Here's how the part is built. I have some questions about the finished solid (model axes, mm). A direction names the side the tool comes from. Coordinates: 2 decimals unless noted, no trailing zeros. Write each loop counter-clockwise with the first axis right and the second up, starting at its lowest first coordinate (ties: lowest second). Pieces come first, ordered by that corner, then holes.
```python
from build123d import *

# Parameters (mm, degrees)
SKETCH_1_R                  = 100
SKETCH_1_W                  = 200
SKETCH_1_H                  = 40
EXTRUDE_524_DEPTH           = 3
SKETCH_3_W                  = 30
SKETCH_3_H                  = 40
SKETCH_3_W_2                = 20
SKETCH_3_H_2                = 30
SKETCH_3_H_3                = 10
CUT_EXTRUDE_1393_DEPTH      = 3
SKETCH_2_R                  = 2
SKETCH_2_R_2                = 1.5
CUT_EXTRUDE_2567_DEPTH      = 173.072659072
REVOLVE_3158_ANGLE          = 90
EXTRUDE_3359_DEPTH          = 40
SKETCH_8_W                  = 10
SKETCH_8_H                  = 8
EXTRUDE_L_DEPTH             = 100
EXTRUDE_L_32_DEPTH          = 10
SKETCH_16_W                 = 2
SKETCH_16_H                 = 84
CUT_EXTRUDE_L_DEPTH         = 5
SKETCH_23_W                 = 200
SKETCH_23_H                 = 3
EXTRUDE_5603_DEPTH          = 100
CUT_EXTRUDE_5983_DEPTH      = 100
CUT_EXTRUDE_5983_DEPTH_BACK = 100
CUT_EXTRUDE_6828_DEPTH      = 100


# Read off the part's stored shape, not the designer's step: the extrude step
with BuildPart() as part:
    # Sketch 1 → Extrude 524 (new body)
    with BuildSketch(Plane(origin=(0, 0, 0), x_dir=(1, 0, 0), z_dir=(0, 1, 0))):
        Circle(SKETCH_1_R)
        with Locations((0, 40)):
            Circle(SKETCH_1_R)
        with Locations((0, 20)):
            Rectangle(SKETCH_1_W, SKETCH_1_H)
    extrude(amount=EXTRUDE_524_DEPTH)

    # Sketch 3 → Cut-Extrude 1393 (cut)
    with BuildSketch(Plane(origin=(0, 3, 0), x_dir=(1, 0, 0), z_dir=(0, 1, 0))):
        with Locations((-79, 20)):
            Rectangle(SKETCH_3_W, SKETCH_3_H)
        with Locations((79, 20)):
            Rectangle(SKETCH_3_W, SKETCH_3_H)
        with Locations((0, -52)):
            Rectangle(SKETCH_3_W_2, SKETCH_3_H_2)
        with Locations((-45, 65)):
            Rectangle(SKETCH_3_W_2, SKETCH_3_H_3)
        with Locations((45, 65)):
            Rectangle(SKETCH_3_W_2, SKETCH_3_H_3)
    extrude(amount=-CUT_EXTRUDE_1393_DEPTH, mode=Mode.SUBTRACT)

    # Sketch 2 → Cut-Extrude 2567 (cut, through all)
    with BuildSketch(Plane(origin=(0, 3, 0), x_dir=(1, 0, 0), z_dir=(0, 1, 0))):
        with Locations(Location((-88, 66, 0), (0, 0, 270))):
            Circle(SKETCH_2_R)
        with Locations(Location((-26, 66, 0), (0, 0, 270))):
            Circle(SKETCH_2_R)
        with Locations(Location((-26, 114, 0), (0, 0, 270))):
            Circle(SKETCH_2_R)
        with Locations(Location((26, 114, 0), (0, 0, 270))):
            Circle(SKETCH_2_R)
        with Locations(Location((26, 66, 0), (0, 0, 270))):
            Circle(SKETCH_2_R)
        with Locations(Location((88, 66, 0), (0, 0, 270))):
            Circle(SKETCH_2_R)
        with Locations(Location((-45, -22, 0), (0, 0, 270))):
            Circle(SKETCH_2_R)
        with Locations(Location((45, -22, 0), (0, 0, 270))):
            Circle(SKETCH_2_R)
        with Locations(Location((-40, -82, 0), (0, 0, 270))):
            Circle(SKETCH_2_R)
        with Locations(Location((40, -82, 0), (0, 0, 270))):
            Circle(SKETCH_2_R)
        with Locations(Location((-45, 90, 0), (0, 0, 270))):
            Circle(SKETCH_2_R_2)
        with Locations(Location((45, 90, 0), (0, 0, 270))):
            Circle(SKETCH_2_R_2)
    extrude(amount=-CUT_EXTRUDE_2567_DEPTH, mode=Mode.SUBTRACT)

    # Sketch 18 → Revolve 3158 (revolve)
    with BuildSketch(Plane(origin=(0, 3, 0), x_dir=(1, 0, 0), z_dir=(0, 1, 0))):
        with BuildLine():
            Line((-97, 0), (-100, 0))
            ThreePointArc((-100, 0), (0, -100), (100, 0))
            Line((100, 0), (97, 0))
            ThreePointArc((97, 0), (0, -97), (-97, 0))
        make_face()
    revolve(axis=Axis((-100, 3, 0), (-1, 0, 0)), revolution_arc=REVOLVE_3158_ANGLE)

    # Sketch 19 → Extrude 3359 (add)
    with BuildSketch(Plane(origin=(0, 0, 0), x_dir=(-1, 0, 0), z_dir=(0, 0, -1))):
        with BuildLine():
            Line((97, 3), (100, 3))
            ThreePointArc((100, 3), (0, 103), (-100, 3))
            Line((-100, 3), (-97, 3))
            ThreePointArc((-97, 3), (0, 100), (97, 3))
        make_face()
    extrude(amount=EXTRUDE_3359_DEPTH)

    # Sketch 8 → Extrude L (add)
    with BuildSketch(Plane(origin=(0, 3, 0), x_dir=(1, 0, 0), z_dir=(0, 1, 0))):
        with Locations((-55, 0)):
            Rectangle(SKETCH_8_W, SKETCH_8_H)
    extrude_l = extrude(amount=EXTRUDE_L_DEPTH)

    # Sketch 11 → Extrude L-32 (add)
    with BuildSketch(Plane.ZY.offset(60)):
        Polygon((37, 3), (4, 60.15767665), (3.758069686, 76.576712245), (46.237604307, 3), align=None)
    extrude_l_32 = extrude(amount=-EXTRUDE_L_32_DEPTH)

    # Sketch 16 → Cut-Extrude L (cut)
    with BuildSketch(Plane(origin=(-50, 0, 0), x_dir=(0, 0, -1), z_dir=(1, 0, 0))):
        Polygon((-32.464101615, 16.856406461), (-34.196152423, 17.856406461), (15.803847577, 104.458946839), (17.535898385, 103.458946839), align=None)
        with Locations((0, 61)):
            Rectangle(SKETCH_16_W, SKETCH_16_H)
    cut_extrude_l = extrude(amount=-CUT_EXTRUDE_L_DEPTH, mode=Mode.SUBTRACT)

    # Mirror R: Extrude L, Extrude L-32, Cut-Extrude L across plane
    add(extrude_l.mirror(Plane(origin=(0, 0, 0), x_dir=(0, 0, 1), z_dir=(1, 0, 0))))
    add(extrude_l_32.mirror(Plane(origin=(0, 0, 0), x_dir=(0, 0, 1), z_dir=(1, 0, 0))))
    add(cut_extrude_l.mirror(Plane(origin=(0, 0, 0), x_dir=(0, 0, 1), z_dir=(1, 0, 0))), mode=Mode.SUBTRACT)

    # Sketch 23 → Extrude 5603 (add)
    with BuildSketch(Plane(origin=(0, 3, 0), x_dir=(1, 0, 0), z_dir=(0, 1, 0))):
        with Locations((0, 41.5)):
            Rectangle(SKETCH_23_W, SKETCH_23_H)
    extrude(amount=EXTRUDE_5603_DEPTH)

    # Sketch 24 → Cut-Extrude 5983 (cut, two sides: drawn at the far end of the back side and taken through both)
    with BuildSketch(Plane.XY.offset(-40).offset(-CUT_EXTRUDE_5983_DEPTH_BACK)):
        with BuildLine():
            ThreePointArc((0, 153), (-106.066017178, 109.066017178), (-150, 3))
            Line((-150, 3), (-100, 3))
            ThreePointArc((-100, 3), (-70.710678119, 73.710678119), (0, 103))
            Line((0, 103), (100, 103))
            Line((100, 103), (100, 3))
            Line((100, 3), (150, 3))
            ThreePointArc((150, 3), (106.066017178, 109.066017178), (0, 153))
        make_face()
        with BuildLine():
            Line((100, 3), (100, 103))
            Line((100, 103), (0, 103))
            ThreePointArc((0, 103), (70.710678119, 73.710678119), (100, 3))
        make_face()
    extrude(amount=CUT_EXTRUDE_5983_DEPTH + CUT_EXTRUDE_5983_DEPTH_BACK, mode=Mode.SUBTRACT)

    # Cut-Extrude 6828 outline → Cut-Extrude 6828 (cut)
    with BuildSketch(Plane(origin=(0, 3, 0), x_dir=(1, 0, 0), z_dir=(0, 1, 0))):
        with BuildLine():
            Line((50, 43), (-50, 43))
            Line((-50, 43), (-50, -50))
            ThreePointArc((-50, -50), (0, -70.710678119), (50, -50))
            Line((50, -50), (50, 43))
        make_face()
    extrude(amount=CUT_EXTRUDE_6828_DEPTH, mode=Mode.SUBTRACT)


solid = part.part
```
1) Imagine slicing it at B-B on z = 17. Please give me the cut outline in (x, y).
Values follow:
outline: (-98.54, 0) - (98.54, 0) - (98.54, 3) arc R98.54 ccw to (50, 87.92) - (50, 84.36) arc R95.5 cw to (95.5, 3) - (-95.5, 3) arc R95.5 cw to (-50, 84.36) - (-50, 87.92) arc R98.54 ccw to (-98.54, 3) - close; (-60, 37.64) - (-50, 37.64) - (-50, 43.64) - (-55, 43.64) - (-55, 47.64) - (-50, 47.64) - (-50, 53.64) - (-60, 53.64) - close; (50, 37.64) - (60, 37.64) - (60, 53.64) - (50, 53.64) - (50, 47.64) - (55, 47.64) - (55, 43.64) - (50, 43.64) - close
2) Imagine slicing it at A-A on x = 0. Please give me the cut outline in (y, z), then the cut area to 3 significant figures.
Values follow:
outline: (0, -140) - (3, -140) - (3, 37) - (0, 37) - close; (0, 67) - (3, 67) - (3, 97) arc R97 cw to (69.4, 70.71) - (73.71, 70.71) arc R100 ccw to (3, 100) - (0, 100) - close
area: 858 mm2
3) I need wall thicknesses on probe 1 along Y at (x, z) = (59, 9); probe 2 along Z at (x, y) = (-55, 13.5); probe 3 along X at (y, z) = (1, -90). Which ranges of each line are inside material? Lowest first, please.
Values follow:
probe 1: y = 0 to 3, 51.5 to 67.5, 79.47 to 83.24
probe 2: z = -43 to -40, -4 to 4, 30.94 to 40.18, 79.21 to 82.85
probe 3: x = -86.6 to -46.5, -43.5 to 43.5, 46.5 to 86.6
4) Will these pins go through, and if not, where does the flat tip stop? pin 1 (5 mm diameter, centred on x = -45, z = -90, fed in from +Y); pin 2 (10.5 mm diameter, centred on y = 65, z = -26, fed in from +X); pin 3 (3 mm diameter, centred on y = 17.5, z = -6, fed in from -X).
Values follow:
pin 1: stops at y = 3
pin 2: stops at x = 82.34
pin 3: stops at x = -99.15
5) We'd pull the mould along Y, two halves only. Please class faces 4 (the face through (-55, 42, -4)), 5 (the face through (-86.97, 52.36, -19.83)), 6 (the face through (-50, 43, 15)): pulls with the +Y half, pulls with the -Y half, needs draft (parallel to the pull), parting line crosses it, or undercut.
Values follow:
face 4: undercut
face 5: pulls with the +Y half
face 6: needs draft
6) Imagine slicing it at C-C on y = 29.5. Count the separate pieces of the cut face and the enclosed holes in it, then the cut area to 3 significant figures.
Values follow:
separate pieces: 5
enclosed holes: 0
area: 1,760 mm2
7) On a 3-axis mill with a long thin cutter (end or side, diameter ignored), from which of +Z, -Z, +X, -X, +Y, -Y can I reach the whole of each face in a straight line? I mean faces 1 (the face through (-52, 82, 1)), 2 (the face through (55.07, 31.18, 20.73)), 3 (the face through (-0.777, 71.525, 70.706)). Say none if no direction works.
Values follow:
face 1: +Y
face 2: none
face 3: -Z, +Y
8) Imagine slicing it at D-D on z = -48. Please give me the cut outline in (x, y), then the cut area to 3 significant figures.
Values follow:
outline: (-99.68, 0) - (99.68, 0) - (99.68, 3) - (-99.68, 3) - close
area: 598 mm2
